Can you work these out from the model? Positions are in its coordinate system, mm. Give positions to 0.01 mm unless a question says otherwise; leave off trailing zeros. Loops run counter-clockwise (first coordinate to the right, second up) from the corner with the lowest first, then second, coordinate; pieces in that order, holes last. Notation, with made-up numbers: (-13.75, 7.25) -> (24.25, 7.25) arc R25 ccw to (24.25, 46.25) -> close; hole circle Ø9 at (27.5, -8). An arc over 180 degrees is marked (long way). One line per question, with ' | ' between items.
from build123d import *

# Parameters (mm, degrees)
BOSS_EXTRUDE1_DEPTH = 16.383
FILLET1_R           = 2


with BuildPart() as part:
    # Sketch1 → Boss-Extrude1 (new, symmetric)
    with BuildSketch(Plane(origin=(0, 0, 0), x_dir=(0, 0, -1), z_dir=(1, 0, 0))):
        with BuildLine():
            Line((-12.5, 56.5), (-12.5, 0))
            Line((-12.5, 0), (12.5, 0))
            Line((12.5, 0), (12.5, 56.5))
            ThreePointArc((12.5, 56.5), (0, 69), (-12.5, 56.5))
        make_face()
    extrude(amount=BOSS_EXTRUDE1_DEPTH, both=True)

    # Fillet1
    fillet1_edges = [part.edges().sort_by_distance(p)[0] for p in [
        (16.383, 0, 0),
        (16.383, 28.25, -12.5),
        (16.383, 69, 0),
        (-16.383, 28.25, -12.5),
        (-16.383, 0, 0),
        (-16.383, 28.25, 12.5),
        (-16.383, 69, 0),
        (0, 0, -12.5),
        (0, 0, 12.5),
        (16.383, 28.25, 12.5),
    ]]
    fillet(fillet1_edges, radius=FILLET1_R)


solid = part.part
Q1. If I drill on probe 1 along Y at (x, z) = (7, 0.25); probe 2 along Z at (x, y) = (-14.5, 47.5); probe 3 along X at (y, z) = (55.5, 10.75), over which ranges is the centre line in solid material (lowest first)? Write a range as from..to.
Entries:
probe 1: 0..69 | probe 2: -12.5..12.5 | probe 3: -16.37..16.37
Q2. If we section it at A-A (x = 13): Write out the boundary of the cut face in (y, z), plus the area to 3 significant figures.
Entries:
outline: (0, -10.5) arc R2 ccw to (2, -12.5) -> (56.5, -12.5) arc R12.5 ccw to (56.5, 12.5) -> (2, 12.5) arc R2 ccw to (0, 10.5) -> close | area: 1,660 mm²
Q3. For pin 1 Ø5 at (x, z) = (-4.5, -3) entering from +Y, with a flat end and sliding along its axis, tell me the tip position at first contact or that it passes through.
Entries:
pin 1: y = 68.99
